Part model, mm, in its own coordinate system. A direction names the side the tool comes from. Give positions to 0.01 mm unless a question says otherwise; leave off trailing zeros. Order: outer loops, then holes, each group sorted by start corner. A loop starts at its lowest first (then second) coordinate and runs counter-clockwise, first axis right, second up. Notation, with made-up numbers: M 89.5,80 L 110.5,80 A27 cw 110.5,106 Z; hole C -3,89.5 d1. An arc over 180 degrees is marked long. Return JSON: item names as keys, results as strings.
from build123d import *

# Parameters (mm, degrees)
SKETCH1_W           = 96.52
SKETCH1_H           = 50.8
BOSS_EXTRUDE1_DEPTH = 5.588
SKETCH2_W           = 61.976
SKETCH2_H           = 50.8
CUT_EXTRUDE2_DEPTH  = 3.048
SKETCH3_W           = 6.35
SKETCH3_H           = 50.8
CUT_EXTRUDE3_DEPTH  = 2.54
SKETCH4_W           = 78.232
SKETCH4_H           = 6.35
BOSS_EXTRUDE2_DEPTH = 17.526
SKETCH5_R           = 2.286
CUT_EXTRUDE4_DEPTH  = 51.8
BOSS_EXTRUDE3_DEPTH = 2.54
BOSS_EXTRUDE4_DEPTH = 2.54
SKETCH8_W           = 6.35
SKETCH8_H           = 8.89
CUT_EXTRUDE5_DEPTH  = 6.588
SKETCH9_W           = 6.35
SKETCH9_H           = 3.048
BOSS_EXTRUDE5_DEPTH = 8.89


with BuildPart() as part:
    # Sketch1 → Boss-Extrude1 (new body)
    with BuildSketch(Plane(origin=(0, 0, 0), x_dir=(1, 0, 0), z_dir=(0, 1, 0))):
        Rectangle(SKETCH1_W, SKETCH1_H)
    extrude(amount=BOSS_EXTRUDE1_DEPTH)

    # Sketch2 → Cut-Extrude2 (cut)
    with BuildSketch(Plane(origin=(0, 5.588, 0), x_dir=(1, 0, 0), z_dir=(0, 1, 0))):
        Rectangle(SKETCH2_W, SKETCH2_H)
    extrude(amount=-CUT_EXTRUDE2_DEPTH, mode=Mode.SUBTRACT)

    # Sketch3 → Cut-Extrude3 (cut)
    with BuildSketch(Plane(origin=(0, 0, 0), x_dir=(-1, 0, 0), z_dir=(0, -1, 0))):
        with Locations((-45.085, 0)):
            Rectangle(SKETCH3_W, SKETCH3_H)
        with Locations((45.085, 0)):
            Rectangle(SKETCH3_W, SKETCH3_H)
    extrude(amount=-CUT_EXTRUDE3_DEPTH, mode=Mode.SUBTRACT)

    # Sketch4 → Boss-Extrude2 (add)
    with BuildSketch(Plane(origin=(0, 2.54, 0), x_dir=(1, 0, 0), z_dir=(0, 1, 0))):
        with Locations((0, 22.225)):
            Rectangle(SKETCH4_W, SKETCH4_H)
    extrude(amount=BOSS_EXTRUDE2_DEPTH)

    # Sketch5 → Cut-Extrude4 (cut, through all)
    with BuildSketch(Plane(origin=(0, 0, -25.4), x_dir=(-1, 0, 0), z_dir=(0, 0, -1))):
        with Locations((13.716, 10.16)):
            Circle(SKETCH5_R)
        with Locations((-13.716, 10.16)):
            Circle(SKETCH5_R)
    extrude(amount=-CUT_EXTRUDE4_DEPTH, mode=Mode.SUBTRACT)

    # Sketch6 → Boss-Extrude3 (add)
    with BuildSketch(Plane.ZY.offset(39.116)):
        Polygon((-19.05, 5.588), (-12.7, 5.588), (-19.05, 20.066), align=None)
    extrude(amount=-BOSS_EXTRUDE3_DEPTH)

    # Sketch7 → Boss-Extrude4 (add)
    with BuildSketch(Plane(origin=(39.116, 0, 0), x_dir=(0, 0, -1), z_dir=(1, 0, 0))):
        Polygon((19.05, 5.588), (19.05, 20.066), (12.7, 5.588), align=None)
    extrude(amount=-BOSS_EXTRUDE4_DEPTH)

    # Sketch8 → Cut-Extrude5 (cut, through all)
    with BuildSketch(Plane(origin=(0, 5.588, 0), x_dir=(1, 0, 0), z_dir=(0, 1, 0))):
        with Locations((45.085, 20.955)):
            Rectangle(SKETCH8_W, SKETCH8_H)
        with Locations((-45.085, 20.955)):
            Rectangle(SKETCH8_W, SKETCH8_H)
    extrude(amount=-CUT_EXTRUDE5_DEPTH, mode=Mode.SUBTRACT)

    # Sketch9 → Boss-Extrude5 (add)
    with BuildSketch(Plane(origin=(0, 0, -16.51), x_dir=(-1, 0, 0), z_dir=(0, 0, -1))):
        with Locations((-45.085, 4.064)):
            Rectangle(SKETCH9_W, SKETCH9_H)
        with Locations((45.085, 4.064)):
            Rectangle(SKETCH9_W, SKETCH9_H)
    extrude(amount=BOSS_EXTRUDE5_DEPTH)


solid = part.part
Q1. 3-axis set-ups, long thin cutter, end or side, ignore diameter. For faces 1 (the flat face through (39.116, 13, -20)), 2 (the flat face through (-30.988, 4, 3)), 3 (the flat face through (41.91, 1, 0)), 4 (the flat face through (-45, 2.54, 0)): which of +Z, -Z, +X, -X, +Y, -Y reach the whole face in a straight line?
Established:
{"face 1": "+Z, -Z, +X, +Y", "face 2": "+Z, +Y", "face 3": "+Z, -Z, +X, -Y", "face 4": "+Z, -Z, -X, -Y"}
Q2. Pin check, flat tips, straight feed: pin 1 (4 mm diameter, centred on x = 13.716, y = 10.16, fed in from +Z); pin 2 (4 mm diameter, centred on y = 10, z = -18.5, fed in from +X); pin 3 (1.5 mm diameter, centred on x = -32, y = 15.5, fed in from +Z); pin 4 (4 mm diameter, centred on x = -25, z = -9, fed in from +Y). Stop position of each tip, or through.
Established:
{"pin 1": "passes through", "pin 2": "stops at x = 39.12", "pin 3": "stops at z = -19.05", "pin 4": "stops at y = 2.54"}
Q3. Band-saw the part on B-B (z = 5.5). Give the cut face in (x, y).
Established:
{"outline": "M -48.26,2.54 L -41.91,2.54 L -41.91,0 L 41.91,0 L 41.91,2.54 L 48.26,2.54 L 48.26,5.59 L 30.99,5.59 L 30.99,2.54 L -30.99,2.54 L -30.99,5.59 L -48.26,5.59 Z"}
Q4. Band-saw the part on D-D (y = 18.75). Give the cut face in (x, z), then the cut area to 3 significant figures.
Established:
{"outline": "M -39.12,-25.4 L 39.12,-25.4 L 39.12,-18.47 L 36.58,-18.47 L 36.58,-19.05 L -36.58,-19.05 L -36.58,-18.47 L -39.12,-18.47 Z", "area": "500 mm²"}
Q5. Two-plate mould, pull along X, no slides. Class faces 5 (the flat face through (-1, 0, 0)), 6 (the flat face through (0, 2.54, 3)), 7 (the flat face through (-48.26, 4, 0)): +X half, -X half, draft (parallel to the pull), parting line (faces both ways), or undercut.
Established:
{"face 5": "draft", "face 6": "undercut", "face 7": "-X half"}
Q6. Band-saw the part on C-C (x = 6). Give the cut face in (y, z).
Established:
{"outline": "M 0,-25.4 L 20.07,-25.4 L 20.07,-19.05 L 2.54,-19.05 L 2.54,25.4 L 0,25.4 Z"}
Q7. Band-saw the part on A-A (y = 10.16). Give the cut face in (x, z), then the cut area to 3 significant figures.
Established:
{"outline": "M -39.12,-25.4 L -16,-25.4 L -16,-19.05 L -36.58,-19.05 L -36.58,-14.71 L -39.12,-14.71 Z; M -11.43,-25.4 L 11.43,-25.4 L 11.43,-19.05 L -11.43,-19.05 Z; M 16,-25.4 L 39.12,-25.4 L 39.12,-14.71 L 36.58,-14.71 L 36.58,-19.05 L 16,-19.05 Z", "area": "461 mm²"}
Q8. Probe line 1 along X through (y, z) = (9.5, -16); line 2 along Y through (x, z) = (43, -9); line 3 along Z through (x, y) = (30, 12.75). List the from-to ranges inside material, lowest first.
Established:
{"line 1": "x = -39.12 to -36.58, 36.58 to 39.12", "line 2": "y = 2.54 to 5.59", "line 3": "z = -25.4 to -19.05"}
